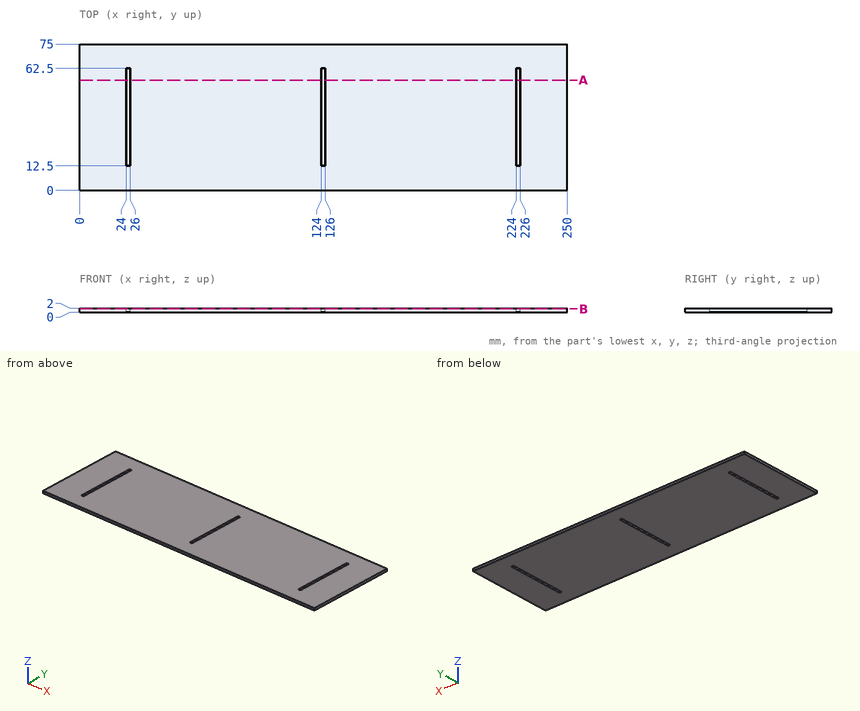
Geometry check sheet. Reference: drawing and pictorial views, mm from the part's lowest x, y, z. Round coordinates to 2 decimals unless told otherwise and drop trailing zeros. Loops run counter-clockwise (first coordinate to the right, second up) from the corner with the lowest first, then second, coordinate; pieces in that order, holes last. Notation, with made-up numbers: (-9.5, 13.25) - (27.5, 13.25) arc R15 ccw to (27.5, 24.25) - close; hole circle Ø6 at (-20, 53). An arc over 180 degrees is marked (long way). One line per question, with ' | ' between items. Start each with the question number.
1. Cross-section at A-A on y = 56.5. Record the cut outline in (x, z), then the cut area to 3 significant figures.
2. Scan lines: line 1 (X direction, y = 44.5, z = 0.35); line 2 (Y direction, x = 224.5, z = 1.45). Record each from-to range of solid material in increasing order. Write a range as [from, to].
3. Cross-section at B-B on z = 1.65. Record the cut outline in (x, y), then the cut area to 4 significant figures.
Taken from the geometry:
1) outline: (0, 0) - (24, 0) - (24, 2) - (0, 2) - close; (26, 0) - (124, 0) - (124, 2) - (26, 2) - close; (126, 0) - (224, 0) - (224, 2) - (126, 2) - close; (226, 0) - (250, 0) - (250, 2) - (226, 2) - close | area: 488 mm²
2) line 1: [0, 24], [26, 124], [126, 224], [226, 250] | line 2: [0, 12.5], [62.5, 75]
3) outline: (0, 0) - (250, 0) - (250, 75) - (0, 75) - close; hole (24, 12.5) - (26, 12.5) - (26, 62.5) - (24, 62.5) - close; hole (124, 12.5) - (126, 12.5) - (126, 62.5) - (124, 62.5) - close; hole (224, 12.5) - (226, 12.5) - (226, 62.5) - (224, 62.5) - close | area: 18,450 mm²
